```python
from build123d import *

# Parameters (mm, degrees)
SKETCH5_W           = 16
SKETCH5_H           = 16
SKETCH5_R           = 2.55
BOSS_EXTRUDE1_DEPTH = 1.75
BOSS_EXTRUDE2_START = 1.75
SKETCH5_4_W         = 16
SKETCH5_4_H         = 16
BOSS_EXTRUDE2_DEPTH = 1.5
BOSS_EXTRUDE3_START = 3.25
SKETCH5_5_R         = 2.25
BOSS_EXTRUDE3_DEPTH = 2.1
BOSS_EXTRUDE4_START = 5.35
SKETCH5_6_R         = 3
SKETCH5_6_R_2       = 2.25
BOSS_EXTRUDE4_DEPTH = 2.25
FILLET1_R           = 1


with BuildPart() as part:
    # Sketch5 → Boss-Extrude1 (new body)
    with BuildSketch(Plane.XY.offset(9.6)):
        with Locations((-64, -16)):
            Rectangle(SKETCH5_W, SKETCH5_H)
        with Locations(Location((-68, -20, 0), (0, 0, 270))):
            Circle(SKETCH5_R, mode=Mode.SUBTRACT)
        with Locations(Location((-60, -20, 0), (0, 0, 270))):
            Circle(SKETCH5_R, mode=Mode.SUBTRACT)
        with Locations(Location((-68, -12, 0), (0, 0, 270))):
            Circle(SKETCH5_R, mode=Mode.SUBTRACT)
        with Locations(Location((-60, -12, 0), (0, 0, 270))):
            Circle(SKETCH5_R, mode=Mode.SUBTRACT)
    extrude(amount=BOSS_EXTRUDE1_DEPTH)

    # Sketch5<4> → Boss-Extrude2 (add)
    with BuildSketch(Plane.XY.offset(9.6).offset(BOSS_EXTRUDE2_START)):
        with Locations((-64, -16)):
            Rectangle(SKETCH5_4_W, SKETCH5_4_H)
    extrude(amount=BOSS_EXTRUDE2_DEPTH)

    # Sketch5<5> → Boss-Extrude3 (add)
    with BuildSketch(Plane.XY.offset(9.6).offset(BOSS_EXTRUDE3_START)):
        with BuildLine():
            Line((-66.969743255, -8), (-72, -8))
            Line((-72, -8), (-72, -24))
            Line((-72, -24), (-66.94438024, -24))
            ThreePointArc((-66.94438024, -24), (-64, -26.425), (-61.05561976, -24))
            Line((-61.05561976, -24), (-56, -24))
            Line((-56, -24), (-56, -8))
            Line((-56, -8), (-61.030256745, -8))
            ThreePointArc((-61.030256745, -8), (-64, -5.425), (-66.969743255, -8))
        make_face()
        with Locations(Location((-64, -23.425, 0), (0, 0, 194.806506912))):
            Circle(SKETCH5_5_R, mode=Mode.SUBTRACT)
        with Locations(Location((-64, -8.425, 0), (0, 0, 169.11205187))):
            Circle(SKETCH5_5_R, mode=Mode.SUBTRACT)
    extrude(amount=BOSS_EXTRUDE3_DEPTH)

    # Sketch5<6> → Boss-Extrude4 (add)
    # profile 1 of 2: a face of its own
    with BuildSketch(Plane.XY.offset(9.6).offset(BOSS_EXTRUDE4_START)):
        with Locations(Location((-64, -8.425, 0), (0, 0, 171.855699446))):
            Circle(SKETCH5_6_R)
        with Locations(Location((-64, -8.425, 0), (0, 0, 169.11205187))):
            Circle(SKETCH5_6_R_2, mode=Mode.SUBTRACT)
    # profile 2 of 2: a face of its own
    with BuildSketch(Plane.XY.offset(9.6).offset(BOSS_EXTRUDE4_START)):
        with Locations(Location((-64, -23.425, 0), (0, 0, 191.050064959))):
            Circle(SKETCH5_6_R)
        with Locations(Location((-64, -23.425, 0), (0, 0, 194.806506912))):
            Circle(SKETCH5_6_R_2, mode=Mode.SUBTRACT)
    extrude(amount=BOSS_EXTRUDE4_DEPTH)

    # Fillet1
    # the kernel refuses this fillet: 1 mm, written as the material it adds along each edge
    with BuildSketch(Plane(origin=(-64, -8.425, 14.95), x_dir=(-0.5594516759376825, 0.8288629695495621, 0), z_dir=(0.8288629695495621, 0.5594516759376825, 0))) as fillet1_piece_1_section:
        with BuildLine():
            CenterArc((3 + FILLET1_R, FILLET1_R), FILLET1_R, 180, 90)
            Line((3, FILLET1_R), (3, 0))
            Line((3, 0), (3 + FILLET1_R, 0))
        make_face()
    fillet1_piece_1 = revolve(axis=Axis((-64, -8.425, 14.95), (0, 0, 1)), revolution_arc=291.964228084, mode=Mode.PRIVATE)
    fillet1_piece_1 = split(fillet1_piece_1, bisect_by=Plane(origin=(-64, -8, 15.233484072), z_dir=(0, -1, 0)), keep=Keep.TOP, mode=Mode.PRIVATE)
    add(fillet1_piece_1)
    with BuildSketch(Plane(origin=(-64, -23.425, 14.95), x_dir=(0.516632343586421, -0.8562073472941015, 0), z_dir=(-0.8562073472941015, -0.516632343586421, 0))) as fillet1_piece_2_section:
        with BuildLine():
            CenterArc((3 + FILLET1_R, FILLET1_R), FILLET1_R, 180, 90)
            Line((3 + FILLET1_R, 0), (3, 0))
            Line((3, 0), (3, FILLET1_R))
        make_face()
    fillet1_piece_2 = revolve(axis=Axis((-64, -23.425, 14.95), (0, 0, 1)), revolution_arc=297.786748706, mode=Mode.PRIVATE)
    fillet1_piece_2 = split(fillet1_piece_2, bisect_by=Plane(origin=(-64, -24, 15.23339809), z_dir=(0, 1, 0)), keep=Keep.TOP, mode=Mode.PRIVATE)
    add(fillet1_piece_2)
    with BuildSketch(Plane(origin=(-58.55561976, -24, 12.85), x_dir=(0, 0, -1), z_dir=(-1, 0, 0))) as fillet1_piece_3_section:
        with BuildLine():
            CenterArc((FILLET1_R, FILLET1_R), FILLET1_R, 180, 90)
            Line((0, FILLET1_R), (0, 0))
            Line((0, 0), (FILLET1_R, 0))
        make_face()
    fillet1_piece_3 = extrude(amount=5.769092903, mode=Mode.PRIVATE)
    fillet1_piece_3 = fillet1_piece_3 - Plane(origin=(-64, -23.425, 12.629693614), x_dir=(-0.9667943721514972, -0.2555555555572849, 0), z_dir=(0, 0, -1)) * Cylinder(2.25, 16, mode=Mode.PRIVATE)
    fillet1_piece_3 = fillet1_piece_3 & Plane(origin=(-64, -23.425, 12.629693614), x_dir=(-0.9814600801300545, -0.19166666666665624, 0), z_dir=(0, 0, -1)) * Cylinder(3, 16, mode=Mode.PRIVATE)
    add(fillet1_piece_3)
    with BuildSketch(Plane(origin=(-63.675287337, -24, 12.85), x_dir=(0, 0, -1), z_dir=(-1, 0, 0))) as fillet1_piece_4_section:
        with BuildLine():
            CenterArc((FILLET1_R, FILLET1_R), FILLET1_R, 180, 90)
            Line((0, FILLET1_R), (0, 0))
            Line((0, 0), (FILLET1_R, 0))
        make_face()
    fillet1_piece_4 = extrude(amount=5.769092903, mode=Mode.PRIVATE)
    fillet1_piece_4 = fillet1_piece_4 - Plane(origin=(-64, -23.425, 12.629693822), x_dir=(-0.9667943721514972, -0.2555555555572849, 0), z_dir=(0, 0, -1)) * Cylinder(2.25, 16, mode=Mode.PRIVATE)
    fillet1_piece_4 = fillet1_piece_4 & Plane(origin=(-64, -23.425, 12.629693822), x_dir=(-0.9814600801300545, -0.19166666666665624, 0), z_dir=(0, 0, -1)) * Cylinder(3, 16, mode=Mode.PRIVATE)
    add(fillet1_piece_4)
    with BuildSketch(Plane(origin=(-64.290503451, -8, 12.85), x_dir=(0, 1, 0), z_dir=(1, 0, 0))) as fillet1_piece_5_section:
        with BuildLine():
            CenterArc((FILLET1_R, -FILLET1_R), FILLET1_R, 90, 90)
            Line((0, -FILLET1_R), (0, 0))
            Line((0, 0), (FILLET1_R, 0))
        make_face()
    fillet1_piece_5 = extrude(amount=5.760246706, mode=Mode.PRIVATE)
    fillet1_piece_5 = fillet1_piece_5 & Plane(origin=(-64, -8.425, 12.629046525), x_dir=(0.9899144182986506, 0.14166666666666652, 0), z_dir=(0, 0, -1)) * Cylinder(3, 16, mode=Mode.PRIVATE)
    fillet1_piece_5 = fillet1_piece_5 - Plane(origin=(-64, -8.425, 12.629046525), x_dir=(-0.9819984662183027, 0.1888888888868298, 0), z_dir=(0, 0, -1)) * Cylinder(2.25, 16, mode=Mode.PRIVATE)
    add(fillet1_piece_5)
    with BuildSketch(Plane(origin=(-69.469743255, -8, 12.85), x_dir=(0, 1, 0), z_dir=(1, 0, 0))) as fillet1_piece_6_section:
        with BuildLine():
            CenterArc((FILLET1_R, -FILLET1_R), FILLET1_R, 90, 90)
            Line((0, -FILLET1_R), (0, 0))
            Line((0, 0), (FILLET1_R, 0))
        make_face()
    fillet1_piece_6 = extrude(amount=5.760246706, mode=Mode.PRIVATE)
    fillet1_piece_6 = fillet1_piece_6 & Plane(origin=(-64, -8.425, 12.629046589), x_dir=(0.9899144182986506, 0.14166666666666652, 0), z_dir=(0, 0, -1)) * Cylinder(3, 16, mode=Mode.PRIVATE)
    fillet1_piece_6 = fillet1_piece_6 - Plane(origin=(-64, -8.425, 12.629046589), x_dir=(-0.9819984662183027, 0.1888888888868298, 0), z_dir=(0, 0, -1)) * Cylinder(2.25, 16, mode=Mode.PRIVATE)
    add(fillet1_piece_6)


solid = part.part
```
The listing builds one solid part. Answer for the finished solid, in the listing's coordinates (mm). A direction names the side the tool comes from. Coordinates: 2 decimals unless noted, no trailing zeros. Loops run counter-clockwise (first coordinate to the right, second up) from the corner with the lowest first, then second, coordinate; pieces in that order, holes last. Notation, with made-up numbers: M -26,39 L -1,39 A38 ccw -1,77 Z; hole C -35.75,-39 d7. An arc over 180 degrees is marked long. Answer as a JSON object with one key per item and string values. Group by question number.
Item 1: Consider L1, parallel to X at y = -12, z = 10; L2, parallel to X at y = -22, z = 10; L3, parallel to Y at x = -64.5, z = 14.25. Determine where each line is inside the solid, lowest interval first.
Item 2: Determine the mould class of faces 1 (the face through (-61.517, -7.699, 12.565)), 2 (the face through (-64, -26, 12.85)), 3 (the face through (-59.888, -17.452, 10.463)) for opening direction Y: +Y half, -Y half, draft (parallel to the pull), parting line (faces both ways), or undercut.
Item 3: Section B-B (z = 16.5) is taken. Give the number of separate pieces and of enclosed holes in the cut face, and give its area (3 significant figures).
Item 4: Section D-D (x = -59.75) is taken. Write down the section's boundary in (y, z).
Item 5: Which of the six approach directions +Z, -Z, +X, -X, +Y, -Y give full straight-line access (tool end or side, diameter ignored) to faces 4 (the face through (-61.566, -24.301, 12.565)), 5 (the face through (-64, -6, 12.85)), 6 (the face through (-66.3, -18.1, 10.5)), 7 (the face through (-64, -16, 14.95))?
Item 6: Each of these flat-tipped pins is pushed along its axis until it touches: P1, Ø1.3, axis at x = -63, y = -9, coming from the +Z side; P2, Ø2.5, axis at x = -59, y = -20.5, coming from the -Z side; P3, Ø3, axis at x = -69.5, z = 10.5, coming from the -Y side. Where does it stop, or does it pass through?
Item 7: Section A-A (x = -64) is taken. Write down the section's boundary in (y, z) (3 decimals).
Solved:
{
 "1": {"L1": "x = -72 to -70.55, -65.45 to -62.55, -57.45 to -56", "L2": "x = -72 to -69.58, -66.42 to -61.58, -58.42 to -56", "L3": "y = -26.38 to -25.62, -21.23 to -10.62, -6.23 to -5.47"},
 "2": {"face 1": "+Y half", "face 2": "draft", "face 3": "undercut"},
 "3": {"separate pieces": "2", "enclosed holes": "2", "area": "24.7 mm2"},
 "4": {"outline": "M -24,9.6 L -22.54,9.6 L -22.54,11.35 L -17.46,11.35 L -17.46,9.6 L -14.54,9.6 L -14.54,11.35 L -9.46,11.35 L -9.46,9.6 L -8,9.6 L -8,14.95 L -24,14.95 Z"},
 "5": {"face 4": "-Z, +X, -X, -Y", "face 5": "-Z, +X, -X, +Y", "face 6": "-Z", "face 7": "+Z"},
 "6": {"P1": "stops at z = 12.85", "P2": "stops at z = 11.35", "P3": "stops at y = -24"},
 "7": {"outline": "M -26.425,12.85 L -25.675,12.85 L -25.675,17.2 L -26.425,17.2 Z; M -24,9.6 L -8,9.6 L -8,12.85 L -10.675,12.85 L -10.675,17.2 L -11.425,17.2 L -11.425,15.95 A1 cw -12.425,14.95 L -19.425,14.95 A1 cw -20.425,15.95 L -20.425,17.2 L -21.175,17.2 L -21.175,12.85 L -24,12.85 Z; M -6.175,12.85 L -5.425,12.85 L -5.425,17.2 L -6.175,17.2 Z"}
}
